For this review, take the finished solid that the model builds, in its own axes (mm). A direction names the side the tool comes from. Coordinates: 2 decimals unless noted, no trailing zeros. Loops run counter-clockwise (first coordinate to the right, second up) from the corner with the lowest first, then second, coordinate; pieces in that order, holes last.
```python
from build123d import *

# Parameters (mm, degrees)
SKETCH1_R           = 20
SKETCH1_R_2         = 3.125
BOSS_EXTRUDE1_DEPTH = 7.5
CUT_EXTRUDE1_START  = -4
SKETCH2_R           = 16.5
SKETCH2_R_2         = 5
CUT_EXTRUDE1_DEPTH  = 37.015621187


with BuildPart() as part:
    # Sketch1 → Boss-Extrude1 (new, symmetric)
    with BuildSketch(Plane(origin=(0, 0, 0), x_dir=(0, 0, -1), z_dir=(1, 0, 0))):
        Circle(SKETCH1_R)
        Circle(SKETCH1_R_2, mode=Mode.SUBTRACT)
    extrude(amount=BOSS_EXTRUDE1_DEPTH, both=True)

    # Sketch2 → Cut-Extrude1 (cut)
    with BuildSketch(Plane(origin=(7.5, 0, 0), x_dir=(0, 0, -1), z_dir=(1, 0, 0)).offset(CUT_EXTRUDE1_START)):
        with Locations(Location((0, 0, 0), (0, 0, 180))):
            Circle(SKETCH2_R)
        with Locations(Location((0, 0, 0), (0, 0, 180))):
            Circle(SKETCH2_R_2, mode=Mode.SUBTRACT)
    cut_extrude1 = extrude(amount=CUT_EXTRUDE1_DEPTH, mode=Mode.SUBTRACT)

    # Mirror1: Cut-Extrude1 across plane
    add(cut_extrude1.mirror(Plane(origin=(0, 0, 0), x_dir=(0, 0, 1), z_dir=(1, 0, 0))), mode=Mode.SUBTRACT)

    # Sketch3 → Cut-Revolve2 (revolve, cut)
    with BuildSketch(Plane.XY, mode=Mode.PRIVATE) as cut_revolve2_sk:
        Polygon((-3.5, 20), (0, 16.5), (3.5, 20), align=None)
    revolve(cut_revolve2_sk.sketch.rotate(Axis((0, 0, 0), (1, 0, 0)), 90), axis=Axis((0, 0, 0), (1, 0, 0)), mode=Mode.SUBTRACT)


solid = part.part
```
Q1. For pin 1 Ø1 at (x, z) = (-0.5, 11.5) entering from -Y; pin 2 Ø1.5 at (y, z) = (-1.5, 9.5) entering from +X; pin 3 Ø2 at (x, y) = (-1.5, -7) entering from -Z, all flat-tipped, find the tip position at first contact; note any pin that passes through.
Q2. The part is to be moulded in two halves that separate along Y. For faces 6 (the face through (5.528, -19.524, 4.336)), 7 (the face through (-3.5, 3.4, -3.9)), 8 (the face through (-7.5, -3.3, 0.1)), say which applies: +Y half, -Y half, draft (parallel to the pull), parting line (faces both ways), or undercut.
Q3. Consider section D-D (x = -0.75). State the section outline as (y, z) points (3 decimals), then the cut area to 3 significant figures.
Q4. Machinability: for faces 1 (the face through (-5.472, -19.524, 4.336)), 2 (the face through (-0.17, 16.274, -3.614)), 3 (the face through (7.5, 16.4, -2.9)), 4 (the face through (-5, 0, -5)), 5 (the face through (5.472, -4.956, 15.738)), which of the approach directions +Z, -Z, +X, -X, +Y, -Y give a long, thin tool a straight path to every point of the face, cutting with its end or side? Answer none if there is none.
Q5. Wall thickness on probe 1 along Y at (x, z) = (-4.4, 0) (3 decimals); probe 2 along Y at (x, z) = (4.25, 2); probe 3 along X at (y, z) = (12.5, 10.5): over which ranges is each line inside the solid? List them lowest first.
Q6. Consider section C-C (x = 4.5). State the section outline as (y, z) points (3 decimals), then the cut area to 3 significant figures.
Model answer:
1. pin 1: stops at y = -13.32
1. pin 2: stops at x = 3.5
1. pin 3: stops at z = -17.73
2. face 6: parting line
2. face 7: undercut
2. face 8: draft
3. outline: circle Ø34.5 at (0, 0); hole circle Ø6.25 at (0, 0)
3. area: 904 mm2
4. face 1: +X, -X
4. face 2: none
4. face 3: +Z, -Z, +X, +Y, -Y
4. face 4: -X
4. face 5: +X
5. probe 1: y = -20 to -16.5, -5 to -3.125, 3.125 to 5, 16.5 to 20
5. probe 2: y = -19.9 to -16.38, -4.58 to -2.4, 2.4 to 4.58, 16.38 to 19.9
5. probe 3: x = -3.5 to 3.5
6. outline: circle Ø40 at (0, 0); circle Ø10 at (0, 0); hole circle Ø33 at (0, 0); hole circle Ø6.25 at (0, 0)
6. area: 449 mm2
